Geometry check sheet. Reference: the model listing, model coordinates, mm. Give positions to 0.01 mm unless a question says otherwise; leave off trailing zeros. Loops run counter-clockwise (first coordinate to the right, second up) from the corner with the lowest first, then second, coordinate; pieces in that order, holes last. Notation, with made-up numbers: (-2.75, 44) -> (14.25, 44) arc R20 cw to (14.25, 71) -> close; hole circle Ø4 at (-23, 74). An arc over 180 degrees is marked (long way). Answer in a Markdown table with one row per item. Add a question column.
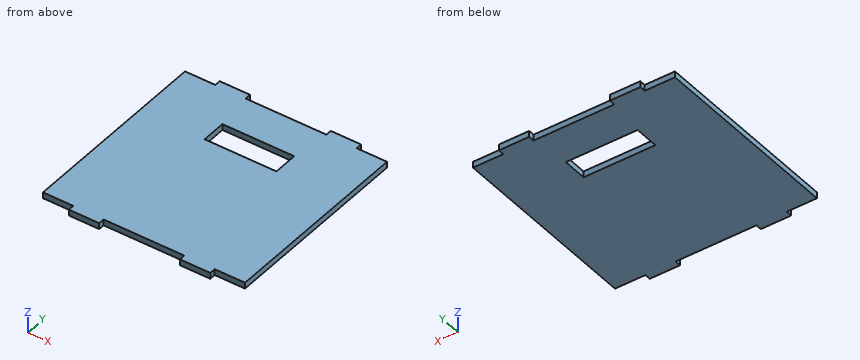
```python
from build123d import *

# Parameters (mm, degrees)
RESSALTO_EXTRUS_O1_DEPTH = 6
ESBO_O4_W                = 71.1
ESBO_O4_H                = 24.3
CORTE_EXTRUS_O2_DEPTH    = 6


with BuildPart() as part:
    # Esboço1 → Ressalto-extrusão1 (new body)
    with BuildSketch(Plane.XY):
        Polygon((-70, -97), (-100, -97), (-100, 97), (-70, 97), (-70, 103), (-40, 103), (-40, 97), (40, 97), (40, 103), (70, 103), (70, 97), (100, 97), (100, -97), (70, -97), (70, -103), (40, -103), (40, -97), (-40, -97), (-40, -103), (-70, -103), align=None)
    extrude(amount=RESSALTO_EXTRUS_O1_DEPTH)

    # Esboço4 → Corte-extrusão2 (cut)
    with BuildSketch(Plane(origin=(0, 0, 0), x_dir=(-1, 0, 0), z_dir=(0, 0, -1))):
        with Locations((0, 47)):
            Rectangle(ESBO_O4_W, ESBO_O4_H)
    extrude(amount=-CORTE_EXTRUS_O2_DEPTH, mode=Mode.SUBTRACT)


solid = part.part
```
1. Material ranges on L1, parallel to X at y = 54, z = 0.65; L2, parallel to Y at x = -3, z = 3.7; L3, parallel to Y at x = -91.5, z = 3.6, recorded low to high. Write a range as from..to.
2. Gauge pin test, flat ends, axial feed: pin 1 Ø3 at (y, z) = (100.5, 2) entering from +X; pin 2 Ø3 at (x, z) = (-14, 2) entering from +Y; pin 3 Ø3 at (x, z) = (19, 4.5) entering from -Y. Record the tip position at first contact, or that the pin passes through.
3. Sectioned sample at A-A (x = -8). Enter the section's corners in (y, z).
4. Sectioned sample at B-B (y = 56.5). Enter the section's corners in (x, z).
5. Sectioned sample at C-C (z = 3.35). Enter the section's corners in (x, y).
Response:
| question | item | result |
|---|---|---|
| 1 | L1 | x = -100..-35.55, 35.55..100 |
| 1 | L2 | y = -97..34.85, 59.15..97 |
| 1 | L3 | y = -97..97 |
| 2 | pin 1 | stops at x = 70 |
| 2 | pin 2 | stops at y = 97 |
| 2 | pin 3 | stops at y = -97 |
| 3 | outline | (-97, 0) -> (34.85, 0) -> (34.85, 6) -> (-97, 6) -> close; (59.15, 0) -> (97, 0) -> (97, 6) -> (59.15, 6) -> close |
| 4 | outline | (-100, 0) -> (-35.55, 0) -> (-35.55, 6) -> (-100, 6) -> close; (35.55, 0) -> (100, 0) -> (100, 6) -> (35.55, 6) -> close |
| 5 | outline | (-100, -97) -> (-70, -97) -> (-70, -103) -> (-40, -103) -> (-40, -97) -> (40, -97) -> (40, -103) -> (70, -103) -> (70, -97) -> (100, -97) -> (100, 97) -> (70, 97) -> (70, 103) -> (40, 103) -> (40, 97) -> (-40, 97) -> (-40, 103) -> (-70, 103) -> (-70, 97) -> (-100, 97) -> close; hole (-35.55, 34.85) -> (35.55, 34.85) -> (35.55, 59.15) -> (-35.55, 59.15) -> close |
